Work out the finished part from the listing and answer in its coordinate system (mm). A direction names the side the tool comes from. Coordinates: 2 decimals unless noted, no trailing zeros. Order: outer loops, then holes, each group sorted by start corner. A loop starts at its lowest first (then second) coordinate and runs counter-clockwise, first axis right, second up. Notation, with made-up numbers: M -10,-24 L 2,-24 A13 ccw 2,1 Z; hole C 78.5,29 d1. An arc over 180 degrees is marked long. Use a Markdown table: item, result. Add a question column.
from build123d import *

# Parameters (mm, degrees)
SKETCH_W        = 130
SKETCH_H        = 104
PAD_DEPTH       = 8
SKETCH001_R     = 2.35
SKETCH001_R_2   = 2.75
POCKET_DEPTH    = 8.001
SKETCH003_R     = 4.6
SKETCH003_W     = 20
SKETCH003_H     = 5
POCKET001_DEPTH = 5
SKETCH002_R     = 1.7
SKETCH002_R_2   = 2.25
SKETCH002_R_3   = 7.5
POCKET002_DEPTH = 8.001
CHAMFER_SIZE    = 3
FILLET_R        = 5


with BuildPart() as part:
    # Sketch → Pad (new body)
    with BuildSketch(Plane.XY):
        Rectangle(SKETCH_W, SKETCH_H)
    extrude(amount=PAD_DEPTH)

    # Sketch001 → Pocket (cut, through all)
    with BuildSketch(Plane.XY.offset(8)):
        with Locations((-35, 46)):
            Circle(SKETCH001_R)
        with Locations((-59, 27)):
            Circle(SKETCH001_R)
        with Locations((-59, 46)):
            Circle(SKETCH001_R)
        with Locations((35, 46)):
            Circle(SKETCH001_R)
        with Locations((59, 28)):
            Circle(SKETCH001_R)
        with Locations((59, 46)):
            Circle(SKETCH001_R)
        with Locations((59, -28)):
            Circle(SKETCH001_R)
        with Locations((59, -46)):
            Circle(SKETCH001_R)
        with Locations((35, -46)):
            Circle(SKETCH001_R)
        with Locations((-59, -28)):
            Circle(SKETCH001_R)
        with Locations((-35, -46)):
            Circle(SKETCH001_R)
        with Locations((-59, -46)):
            Circle(SKETCH001_R)
        with Locations((-47, 46)):
            Circle(SKETCH001_R_2)
        with Locations((-47, 26)):
            Circle(SKETCH001_R_2)
        with Locations((47, 46)):
            Circle(SKETCH001_R_2)
        with Locations((47, 26)):
            Circle(SKETCH001_R_2)
        with Locations((-21, -37)):
            Circle(SKETCH001_R_2)
        with Locations((21, -37)):
            Circle(SKETCH001_R_2)
        with Locations((-21, 37)):
            Circle(SKETCH001_R_2)
        with Locations((21, 37)):
            Circle(SKETCH001_R_2)
        with Locations((47, -46)):
            Circle(SKETCH001_R_2)
        with Locations((47, -26)):
            Circle(SKETCH001_R_2)
        with Locations((-47, -26)):
            Circle(SKETCH001_R_2)
        with Locations((-47, -46)):
            Circle(SKETCH001_R_2)
        with Locations((-35, 28)):
            Circle(SKETCH001_R)
        with Locations((35, 28)):
            Circle(SKETCH001_R)
        with Locations((35, -28)):
            Circle(SKETCH001_R)
        with Locations((-35, -28)):
            Circle(SKETCH001_R)
        with Locations((-59, 9)):
            Circle(SKETCH001_R)
        with Locations((-59, -9)):
            Circle(SKETCH001_R)
        with Locations((-35, 9)):
            Circle(SKETCH001_R)
        with Locations((-35, -9)):
            Circle(SKETCH001_R)
    extrude(amount=-POCKET_DEPTH, mode=Mode.SUBTRACT)

    # Sketch003 → Pocket001 (cut)
    with BuildSketch(Plane(origin=(0, 0, 0), x_dir=(1, 0, 0), z_dir=(0, 0, -1))):
        with Locations((-47, 46)):
            Circle(SKETCH003_R)
        with Locations((47, -26)):
            Circle(SKETCH003_R)
        with Locations((47, 26)):
            Circle(SKETCH003_R)
        with Locations((47, 46)):
            Circle(SKETCH003_R)
        with Locations((-47, 26)):
            Circle(SKETCH003_R)
        with Locations((47, -46)):
            Circle(SKETCH003_R)
        with Locations((-47, -46)):
            Circle(SKETCH003_R)
        with Locations((-47, -26)):
            Circle(SKETCH003_R)
        with Locations((0, -7.279179)):
            Rectangle(SKETCH003_W, SKETCH003_H)
    extrude(amount=-POCKET001_DEPTH, mode=Mode.SUBTRACT)

    # Sketch002 → Pocket002 (cut, through all)
    with BuildSketch(Plane.XY.offset(8)):
        with Locations((-10, 10)):
            Circle(SKETCH002_R)
        with Locations((-20, 10)):
            Circle(SKETCH002_R)
        with Locations((-10, 0)):
            Circle(SKETCH002_R_2)
        with Locations((-20, 0)):
            Circle(SKETCH002_R_2)
        with Locations((-10, -10)):
            Circle(SKETCH002_R)
        with Locations((-20, -10)):
            Circle(SKETCH002_R)
        with Locations((-30, 0)):
            Circle(SKETCH002_R_2)
        with Locations((-40, 0)):
            Circle(SKETCH002_R_2)
        with Locations((10, 10)):
            Circle(SKETCH002_R)
        with Locations((10, -10)):
            Circle(SKETCH002_R)
        with Locations((20, -10)):
            Circle(SKETCH002_R)
        with Locations((20, 10)):
            Circle(SKETCH002_R)
        with Locations((30, 10)):
            Circle(SKETCH002_R)
        with Locations((40, 10)):
            Circle(SKETCH002_R)
        with Locations((30, -10)):
            Circle(SKETCH002_R)
        with Locations((40, -10)):
            Circle(SKETCH002_R)
        with Locations((-10, 20)):
            Circle(SKETCH002_R)
        with Locations((-20, 20)):
            Circle(SKETCH002_R)
        with Locations((10, 20)):
            Circle(SKETCH002_R)
        with Locations((20, 20)):
            Circle(SKETCH002_R)
        with Locations((20, -20)):
            Circle(SKETCH002_R)
        with Locations((10, -20)):
            Circle(SKETCH002_R)
        with Locations((-10, -20)):
            Circle(SKETCH002_R)
        with Locations((-20, -20)):
            Circle(SKETCH002_R)
        with Locations((-10, 30)):
            Circle(SKETCH002_R)
        with Locations((-10, 40)):
            Circle(SKETCH002_R)
        with Locations((10, 40)):
            Circle(SKETCH002_R)
        with Locations((10, 30)):
            Circle(SKETCH002_R)
        with Locations((10, -30)):
            Circle(SKETCH002_R)
        with Locations((-10, -30)):
            Circle(SKETCH002_R)
        with Locations((-10, -40)):
            Circle(SKETCH002_R)
        with Locations((10, -40)):
            Circle(SKETCH002_R)
        with Locations((0, 40)):
            Circle(SKETCH002_R_2)
        with Locations((0, 30)):
            Circle(SKETCH002_R_2)
        with Locations((0, 20)):
            Circle(SKETCH002_R_2)
        with Locations((0, 10)):
            Circle(SKETCH002_R_2)
        with Locations((0, -10)):
            Circle(SKETCH002_R_2)
        with Locations((0, -20)):
            Circle(SKETCH002_R_2)
        with Locations((0, -30)):
            Circle(SKETCH002_R_2)
        with Locations((0, -40)):
            Circle(SKETCH002_R_2)
        with Locations((10, 0)):
            Circle(SKETCH002_R_2)
        with Locations((20, 0)):
            Circle(SKETCH002_R_2)
        with Locations((30, 0)):
            Circle(SKETCH002_R_2)
        with Locations((40, 0)):
            Circle(SKETCH002_R_2)
        with Locations((50, 0)):
            Circle(SKETCH002_R_2)
        with Locations((50, 10)):
            Circle(SKETCH002_R)
        with Locations((50, -10)):
            Circle(SKETCH002_R)
        with Locations((-30, 20)):
            Circle(SKETCH002_R)
        with Locations((-30, -20)):
            Circle(SKETCH002_R)
        with Locations((30, 20)):
            Circle(SKETCH002_R)
        with Locations((30, -20)):
            Circle(SKETCH002_R)
        Circle(SKETCH002_R_3)
    extrude(amount=-POCKET002_DEPTH, mode=Mode.SUBTRACT)

    # Chamfer
    chamfer_edges = [part.edges().sort_by_distance(p)[0] for p in [
        (0, -52, 8),
    ]]
    chamfer(chamfer_edges, length=CHAMFER_SIZE)

    # Fillet
    fillet_edges = [part.edges().sort_by_distance(p)[0] for p in [
        (65, -52, 2.5),
        (65, 52, 4),
        (-65, -52, 2.5),
        (-65, 52, 4),
    ]]
    fillet(fillet_edges, radius=FILLET_R)


solid = part.part
(1) The mould has two halves that part along X. Classify faces 1 (the cylindrical face through (9.63, -31.66, 4.06)), 2 (the cylindrical face through (-64, 50, 4)), 3 (the cylindrical face through (63, -51, 3)), 4 (the cylindrical face through (-44.877, -41.919, 2.465)): pulls with the +X half, pulls with the -X half, needs draft (parallel to the pull), parting line crosses it, or undercut.
(2) Straight lines are drawn through the part: line 1 (X direction, y = -24, z = 6.5); line 2 (Y direction, x = -40, z = 3.5); line 3 (Y direction, x = 3, z = 6). For each, find the intervals that lie inside material, in ascending order.
(3) Which of the six approach directions +Z, -Z, +X, -X, +Y, -Y give full straight-line access (tool end or side, diameter ignored) to faces 5 (the cylindrical face through (58.69, 48.33, 4.06)), 6 (the flat face through (-8, 4.779, 2))?
(4) A cutting plane is placed at A-A on x = 40. Write down the section's boundary in (y, z).
(5) Given P1, Ø5, axis at x = -20, y = 0, coming from the -Z side; P2, Ø4, axis at x = 35, y = -46, coming from the -Z side; P3, Ø9, axis at x = 47, y = 46, coming from the -Z side, each flat-ended and moving along its own axis, determine where each tip first touches the part or whether it passes through.
(6) A cutting plane is placed at B-B on z = 2.25. Count the separate pieces of the cut face and the enclosed holes in it, plus the area to 3 significant figures.
From the geometry:
| question | item | result |
|---|---|---|
| 1 | face 1 | undercut |
| 1 | face 2 | pulls with the -X half |
| 1 | face 3 | pulls with the +X half |
| 1 | face 4 | undercut |
| 2 | line 1 | x = -65 to -48.89, -45.11 to 45.11, 48.89 to 65 |
| 2 | line 2 | y = -52 to -2.25, 2.25 to 52 |
| 2 | line 3 | y = -51 to -6.87, 6.87 to 52 |
| 3 | face 5 | +Z, -Z |
| 3 | face 6 | -Z |
| 4 | outline | M -52,0 L -11.7,0 L -11.7,8 L -49,8 L -52,5 Z; M -8.3,0 L -2.25,0 L -2.25,8 L -8.3,8 Z; M 2.25,0 L 8.3,0 L 8.3,8 L 2.25,8 Z; M 11.7,0 L 52,0 L 52,8 L 11.7,8 Z |
| 5 | P1 | stops at z = 0 |
| 5 | P2 | passes through |
| 5 | P3 | stops at z = 5 |
| 6 | separate pieces | 1 |
| 6 | enclosed holes | 81 |
| 6 | area | 11,700 mm2 |
